Geometry check sheet. Reference: the model listing, model coordinates, mm. A direction names the side the tool comes from. Round coordinates to 2 decimals unless told otherwise and drop trailing zeros. Write each loop counter-clockwise with the first axis right and the second up, starting at its lowest first coordinate (ties: lowest second). Pieces come first, ordered by that corner, then holes.
Item 1: Depth check by flat-ended pin: P1, Ø4, axis at x = 2.5, y = 3, coming from the +Z side; P2, Ø2, axis at x = -4, z = 8.5, coming from the +Y side; P3, Ø1, axis at y = 4, z = 4.5, coming from the +X side. Enter the tip coordinate at first touch or a pass-through.
Item 2: Cross-section at A-A (y = 0). Enter the section's corners in (x, z), then the cut area to 3 significant figures.
Item 3: Access from +Z, -Z, +X, -X, +Y, -Y to the whole of each face (thin tool, end or side, straight path). Record for faces 4 (the face through (5, 3, 0)), 5 (the face through (6.466, -2.681, 12.246)), 6 (the face through (-1.46, -6.59, 9.46)).
Item 4: Cross-section at C-C (z = 4). Enter the section's corners in (x, y), then the cut area to 3 significant figures.
Item 5: Scan lines: probe 1 along Y at (x, z) = (0, 4); probe 2 along X at (y, z) = (-0.25, 13); probe 3 along X at (y, z) = (7.75, 4). Record each from-to range of solid material in increasing order.
Item 6: Cross-section at B-B (x = 0). Enter the section's corners in (y, z).
Item 7: Cross-section at D-D (z = 9.25). Enter the section's corners in (x, y), then the cut area to 3 significant figures.
Item 8: Draft check along Y on faces 1 (the face through (7, -2, 14.5)), 2 (the face through (5, 1.6, 3.5)), 3 (the face through (-2.38, -10.74, 6.66)). Enter one of: pulls with the +Y half, pulls with the -Y half, needs draft (parallel to the pull), parting line crosses it, or undercut.
from build123d import *

# Parameters (mm, degrees)
ESQUISSE1_R                   = 11
ESQUISSE1_R_2                 = 5.25
BOSS_EXTRU_1_DEPTH            = 7
ESQUISSE2_R                   = 11
ESQUISSE2_R_2                 = 6.75
BOSS_EXTRU_2_DEPTH            = 5
ESQUISSE3_R                   = 11
ESQUISSE3_R_2                 = 7
BOSS_EXTRU_3_DEPTH            = 0.5
ESQUISSE4_R                   = 11
ESQUISSE4_R_2                 = 6.75
BOSS_EXTRU_4_DEPTH            = 2
CHANFREIN1_SIZE               = 1
DIAM_TRE_DU_PER_AGE_2_0_2_1_D = 2


with BuildPart() as part:
    # Esquisse1 → Boss.-Extru.1 (new body)
    with BuildSketch(Plane.XY):
        Circle(ESQUISSE1_R)
        Circle(ESQUISSE1_R_2, mode=Mode.SUBTRACT)
    extrude(amount=BOSS_EXTRU_1_DEPTH)

    # Esquisse2 → Boss.-Extru.2 (add)
    with BuildSketch(Plane.XY.offset(7)):
        Circle(ESQUISSE2_R)
        Circle(ESQUISSE2_R_2, mode=Mode.SUBTRACT)
    extrude(amount=BOSS_EXTRU_2_DEPTH)

    # Esquisse3 → Boss.-Extru.3 (add)
    with BuildSketch(Plane.XY.offset(12)):
        Circle(ESQUISSE3_R)
        Circle(ESQUISSE3_R_2, mode=Mode.SUBTRACT)
    extrude(amount=BOSS_EXTRU_3_DEPTH)

    # Esquisse4 → Boss.-Extru.4 (add)
    with BuildSketch(Plane.XY.offset(12.5)):
        Circle(ESQUISSE4_R)
        Circle(ESQUISSE4_R_2, mode=Mode.SUBTRACT)
    extrude(amount=BOSS_EXTRU_4_DEPTH)

    # Chanfrein1
    chanfrein1_edges = [part.edges().sort_by_distance(p)[0] for p in [
        (-11, 0, 14.5),
    ]]
    chamfer(chanfrein1_edges, length=CHANFREIN1_SIZE)

    # Diamètre du perçage Ø2.0 (2)1 (through all)
    with Locations(Plane(origin=(0, 0, 0), x_dir=(-1, 0, 0), z_dir=(0, 0, -1))):
        with Locations((-7.361215932, -4.25), (0, 8.5), (7.361215932, -4.25)):
            Hole(DIAM_TRE_DU_PER_AGE_2_0_2_1_D / 2)


solid = part.part
Resolved:
1. P1: stops at z = 7
1. P2: stops at y = 10.58
1. P3: stops at x = 10.43
2. outline: (-11, 0) - (-5.25, 0) - (-5.25, 7) - (-6.75, 7) - (-6.75, 12) - (-7, 12) - (-7, 12.5) - (-6.75, 12.5) - (-6.75, 14.5) - (-10, 14.5) - (-11, 13.5) - close; (5.25, 0) - (11, 0) - (11, 13.5) - (10, 14.5) - (6.75, 14.5) - (6.75, 12.5) - (7, 12.5) - (7, 12) - (6.75, 12) - (6.75, 7) - (5.25, 7) - close
2. area: 143 mm2
3. face 4: -Z, +X, -X, +Y, -Y
3. face 5: none
3. face 6: +Z
4. outline: circle Ø22 at (0, 0); hole circle Ø2 at (-7.36, -4.25); hole circle Ø10.5 at (0, 0); hole circle Ø2 at (0, 8.5); hole circle Ø2 at (7.36, -4.25)
4. area: 284 mm2
5. probe 1: y = -11 to -5.25, 5.25 to 7.5, 9.5 to 11
5. probe 2: x = -11 to -6.75, 6.75 to 11
5. probe 3: x = -7.81 to -0.66, 0.66 to 7.81
6. outline: (-11, 0) - (-5.25, 0) - (-5.25, 7) - (-6.75, 7) - (-6.75, 12) - (-7, 12) - (-7, 12.5) - (-6.75, 12.5) - (-6.75, 14.5) - (-10, 14.5) - (-11, 13.5) - close; (5.25, 0) - (7.5, 0) - (7.5, 14.5) - (6.75, 14.5) - (6.75, 12.5) - (7, 12.5) - (7, 12) - (6.75, 12) - (6.75, 7) - (5.25, 7) - close; (9.5, 0) - (11, 0) - (11, 13.5) - (10, 14.5) - (9.5, 14.5) - close
7. outline: circle Ø22 at (0, 0); hole circle Ø2 at (-7.36, -4.25); hole circle Ø13.5 at (0, 0); hole circle Ø2 at (0, 8.5); hole circle Ø2 at (7.36, -4.25)
7. area: 228 mm2
8. face 1: needs draft
8. face 2: undercut
8. face 3: parting line crosses it
